from build123d import *

# Parameters (mm, degrees)
SKETCH1_R               = 4
BOSS_EXTRUDE1_DEPTH     = 20
SKETCH2_R               = 3.5
SKETCH2_R_2             = 3.25
CUT_EXTRUDE_THIN1_DEPTH = 0.1
SKETCH3_R               = 2
BOSS_EXTRUDE2_DEPTH     = 0.2
FILLET1_R               = 0.1
SKETCH4_R               = 2
BOSS_EXTRUDE3_DEPTH     = 1
FILLET2_R               = 0.1
SKETCH5_R               = 1.25
BOSS_EXTRUDE4_DEPTH     = 0.5
CHAMFER1_SIZE           = 0.2
BOSS_EXTRUDE5_DEPTH     = 0.25
SKETCH7_R               = 1.5
BOSS_EXTRUDE6_DEPTH     = 10
SKETCH8_R               = 3.5
SKETCH8_R_2             = 3.25
CUT_EXTRUDE_THIN2_DEPTH = 0.1


with BuildPart() as part:
    # Sketch1 → Boss-Extrude1 (new body)
    with BuildSketch(Plane(origin=(0, 0, 0), x_dir=(1, 0, 0), z_dir=(0, 1, 0))):
        Circle(SKETCH1_R)
    extrude(amount=BOSS_EXTRUDE1_DEPTH)

    # Sketch2 → Cut-Extrude-Thin1 (cut)
    with BuildSketch(Plane.XZ):
        Circle(SKETCH2_R)
        Circle(SKETCH2_R_2, mode=Mode.SUBTRACT)
    extrude(amount=-CUT_EXTRUDE_THIN1_DEPTH, mode=Mode.SUBTRACT)

    # Sketch3 → Boss-Extrude2 (add)
    with BuildSketch(Plane.XZ):
        Circle(SKETCH3_R)
    extrude(amount=BOSS_EXTRUDE2_DEPTH)

    # Fillet1
    fillet1_edges = [part.edges().sort_by_distance(p)[0] for p in [
        (-2, -0.2, 0),
    ]]
    fillet(fillet1_edges, radius=FILLET1_R)

    # Sketch4 → Boss-Extrude3 (add)
    with BuildSketch(Plane.XZ.offset(0.2)):
        Circle(SKETCH4_R)
    extrude(amount=BOSS_EXTRUDE3_DEPTH)

    # Fillet2
    fillet2_edges = [part.edges().sort_by_distance(p)[0] for p in [
        (-2, -1.2, 0),
    ]]
    fillet(fillet2_edges, radius=FILLET2_R)

    # Sketch5 → Boss-Extrude4 (add)
    with BuildSketch(Plane.XZ.offset(1.2)):
        Circle(SKETCH5_R)
    extrude(amount=BOSS_EXTRUDE4_DEPTH)

    # Chamfer1
    chamfer1_edges = [part.edges().sort_by_distance(p)[0] for p in [
        (-1.25, -1.7, 0),
    ]]
    chamfer(chamfer1_edges, length=CHAMFER1_SIZE)

    # Sketch6 → Boss-Extrude5 (add)
    with BuildSketch(Plane.XZ.offset(1.2)):
        with BuildLine():
            Line((0, -1.25), (0, -2))
            ThreePointArc((0, -2), (-1.414213562, 1.414213562), (2, 0))
            Line((2, 0), (1.25, 0))
            ThreePointArc((1.25, 0), (-0.883883476, 0.883883476), (0, -1.25))
        make_face()
    extrude(amount=BOSS_EXTRUDE5_DEPTH)

    # Sketch7 → Boss-Extrude6 (add)
    with BuildSketch(Plane(origin=(0, 20, 0), x_dir=(1, 0, 0), z_dir=(0, 1, 0))):
        Circle(SKETCH7_R)
    extrude(amount=BOSS_EXTRUDE6_DEPTH)

    # Sketch8 → Cut-Extrude-Thin2 (cut)
    with BuildSketch(Plane(origin=(0, 20, 0), x_dir=(1, 0, 0), z_dir=(0, 1, 0))):
        Circle(SKETCH8_R)
        Circle(SKETCH8_R_2, mode=Mode.SUBTRACT)
    extrude(amount=-CUT_EXTRUDE_THIN2_DEPTH, mode=Mode.SUBTRACT)


solid = part.part
Input: part model. Units: mm. Frame: model coordinates. A direction names the side the tool comes from. Round coordinates to 2 decimals unless told otherwise and drop trailing zeros. Write each loop counter-clockwise with the first axis right and the second up, starting at its lowest first coordinate (ties: lowest second). Pieces come first, ordered by that corner, then holes.
1) Cut plane A-A (y = 10). Return the cut outline in (x, z).
2) Contact query for flat-ended pins moving along their axis: P1, Ø2, axis at y = 10, z = -2, coming from the -X side; P2, Ø2, axis at x = -0.5, y = 16.5, coming from the +Z side; P3, Ø2, axis at x = 2.5, y = 9, coming from the +Z side. Output: stop coordinate, or through.
3) Cut plane C-C (y = 22.5). Return the cut outline in (x, z).
4) Cut plane B-B (z = -2.5). Return the cut outline in (x, y), then the cut area to 3 significant figures.
5) Reachability of faces 1 (the flat face through (-1.5, 20, 0.7)), 2 (the flat face through (1, 0, 2)), 3 (the flat face through (1, -1.2, -1)), 4 (the flat face through (0, -1.7, 0)) from +Z, -Z, +X, -X, +Y, -Y: full face, straight path, thin tool, end or side. Return the list, or none.
6) Ray query, L1, parallel to Z at x = 0, y = 19.95; L2, parallel to Z at x = 0, y = 20.05; L3, parallel to Y at x = 2.25, z = -0.25. Return the intervals inside material, ascending.
Geometry says:
1. outline: circle Ø8 at (0, 0)
2. P1: stops at x = -3.87
2. P2: stops at z = 4
2. P3: stops at z = 3.71
3. outline: circle Ø3 at (0, 0)
4. outline: (-3.12, 0) - (-2.45, 0) - (-2.45, 0.1) - (-2.08, 0.1) - (-2.08, 0) - (2.08, 0) - (2.08, 0.1) - (2.45, 0.1) - (2.45, 0) - (3.12, 0) - (3.12, 20) - (2.45, 20) - (2.45, 19.9) - (2.08, 19.9) - (2.08, 20) - (-2.08, 20) - (-2.08, 19.9) - (-2.45, 19.9) - (-2.45, 20) - (-3.12, 20) - close
4. area: 125 mm2
5. face 1: +Y
5. face 2: -Y
5. face 3: -Z, +X, -Y
5. face 4: +Z, -Z, +X, -X, -Y
6. L1: z = -4 to -3.5, -3.25 to 3.25, 3.5 to 4
6. L2: z = -1.5 to 1.5
6. L3: y = 0 to 20
